Model file for the job. Use its own axes, mm. A direction names the side the tool comes from. Round coordinates to 2 decimals unless told otherwise and drop trailing zeros. Order: outer loops, then holes, each group sorted by start corner. A loop starts at its lowest first (then second) coordinate and runs counter-clockwise, first axis right, second up. Notation, with made-up numbers: (69, 15.5) - (116, 15.5) arc R38 cw to (116, 54.5) - close; hole circle Ø7 at (83, 8.25). An arc over 180 degrees is marked (long way). Answer as CSV lines item,"result". Start each with the question number.
1. Band-saw the part on D-D on z = -5.25. List the corners of the cut face in (x, y), then the cut area to 3 significant figures.
2. Band-saw the part on B-B on y = 17. List the corners of the cut face in (x, z), then the cut area to 3 significant figures.
3. Band-saw the part on C-C on y = 42. List the corners of the cut face in (x, z), then the cut area to 3 significant figures.
4. Wall check: line 1 along X through (y, z) = (2.1, 0); line 2 along Y through (x, z) = (0, 12.25); line 3 along X through (y, z) = (35, -4.5). Give the ranges that are in metal, low to high. Write a range as [from, to].
5. Pin check, flat tips, straight feed: pin 1 Ø9 at (x, y) = (25, 15) entering from +Z; pin 2 Ø1 at (x, z) = (-12.5, 9) entering from +Y; pin 3 Ø13.5 at (x, z) = (-20, 0) entering from +Y. Stop position of each tip, or through.
6. 3-axis set-ups, long thin cutter, end or side, ignore diameter. For faces 1 (the face through (-1.301, 32.143, 11.521)), 2 (the face through (-35.14, 25.35, 12.1)), 3 (the face through (-8, 3, 0)): which of +Z, -Z, +X, -X, +Y, -Y reach the whole face in a straight line?
7. Band-saw the part on A-A on z = 0. List the corners of the cut face in (x, y).
8. Pull direction Z, two halves, no side cores. Call faces 4 (the face through (0.33, 1.521, -7.493)), 5 (the face through (35.14, 25.35, -12.1)), 6 (the face through (-0.976, 27.436, 11.521)): released by +Z, released by -Z, zero draft, split by the parting line, or undercut.
```python
from build123d import *

# Parameters (mm, degrees)
SKETCH1_W                                    = 72
SKETCH1_H                                    = 26
BOSS_EXTRUDE1_DEPTH                          = 50
FILLET1_R                                    = 3
SHELL1_START                                 = -33
SHELL1_OUTLINE_W                             = 47
SHELL1_OUTLINE_H                             = 20
SHELL1_DEPTH                                 = 66
SKETCH2_R                                    = 7.5
CUT_EXTRUDE1_DEPTH                           = 61.613529843
CSK_FOR_M3_COUNTERSUNK_FLAT_HEAD_SCR_2_COUNT = 2
CSK_FOR_M3_COUNTERSUNK_FLAT_HEAD_SCR_2_PITCH = 30.663496213
CSK_FOR_M3_COUNTERSUNK_FLAT_HEAD_SCR_3_COUNT = 2
CSK_FOR_M3_COUNTERSUNK_FLAT_HEAD_SCR_3_PITCH = 30.663496213
CUT_EXTRUDE2_REACH                           = 68.873
SKETCH6_R                                    = 6
SKETCH6_R_2                                  = 7.5
SKETCH6_R_3                                  = 5


# Read off the part's stored shape, not the designer's step: Shell1
with BuildPart() as part:
    # Sketch1 → Boss-Extrude1 (new body)
    with BuildSketch(Plane(origin=(0, 0, 0), x_dir=(1, 0, 0), z_dir=(0, 1, 0))):
        Rectangle(SKETCH1_W, SKETCH1_H)
    extrude(amount=BOSS_EXTRUDE1_DEPTH)

    # Fillet1
    fillet1_edges = [part.edges().sort_by_distance(p)[0] for p in [
        (-36, 25, -13),
        (36, 25, -13),
        (36, 25, 13),
        (-36, 25, 13),
    ]]
    fillet(fillet1_edges, radius=FILLET1_R)

    # Shell1 outline → Shell1 (cut)
    with BuildSketch(Plane.YZ.offset(SHELL1_START)):
        with Locations((26.5, 0)):
            Rectangle(SHELL1_OUTLINE_W, SHELL1_OUTLINE_H)
    extrude(amount=SHELL1_DEPTH, mode=Mode.SUBTRACT)

    # Sketch2 → Cut-Extrude1 (cut, through all)
    with BuildSketch(Plane(origin=(0, 3, 0), x_dir=(1, 0, 0), z_dir=(0, 1, 0))):
        with Locations(Location((0, 0, 0), (0, 0, 270))):
            Circle(SKETCH2_R)
        with Locations(Location((-20, 0, 0), (0, 0, 270))):
            Circle(SKETCH2_R)
        with Locations(Location((20, 0, 0), (0, 0, 270))):
            Circle(SKETCH2_R)
    extrude(amount=-CUT_EXTRUDE1_DEPTH, mode=Mode.SUBTRACT)

    # Sketch4 → CSK for M3 Countersunk Flat Head Screw1 (revolve, cut)
    with BuildSketch(Plane(origin=(0, 38, -10), x_dir=(0, -1, 0), z_dir=(1, 0, 0))):
        Polygon((0, 0), (0, 3), (1.7, 3), (1.7, 1.45), (3.15, 0), align=None)
    csk_for_m3_countersunk_flat_head_screw1 = revolve(axis=Axis((0, 38, -3.65), (0, 0, -1)), mode=Mode.SUBTRACT)

    # CSK for M3 Countersunk Flat Head Scr 2: CSK for M3 Countersunk Flat Head Screw1 ×2
    with Locations(*[Vector(-0.4076508403738889, -0.9131378824375114, 0) * (i * CSK_FOR_M3_COUNTERSUNK_FLAT_HEAD_SCR_2_PITCH) for i in range(1, CSK_FOR_M3_COUNTERSUNK_FLAT_HEAD_SCR_2_COUNT)]):
        add(csk_for_m3_countersunk_flat_head_screw1, mode=Mode.SUBTRACT)

    # CSK for M3 Countersunk Flat Head Scr 3: CSK for M3 Countersunk Flat Head Screw1 ×2
    with Locations(*[Vector(0.4076508403738889, -0.9131378824375114, 0) * (i * CSK_FOR_M3_COUNTERSUNK_FLAT_HEAD_SCR_3_PITCH) for i in range(1, CSK_FOR_M3_COUNTERSUNK_FLAT_HEAD_SCR_3_COUNT)]):
        add(csk_for_m3_countersunk_flat_head_screw1, mode=Mode.SUBTRACT)

    # Sketch6 → Cut-Extrude2 (cut, up to next)
    with BuildSketch(Plane.XY.offset(13), mode=Mode.PRIVATE) as cut_extrude2_sk1:
        with Locations((0, 38)):
            Circle(SKETCH6_R)
    cut_extrude2_tool1 = extrude(cut_extrude2_sk1.sketch, amount=-CUT_EXTRUDE2_REACH, mode=Mode.PRIVATE) & part.part
    # Sketch6 → Cut-Extrude2 (cut, up to next)
    with BuildSketch(Plane.XY.offset(13), mode=Mode.PRIVATE) as cut_extrude2_sk2:
        with Locations((-12.5, 10)):
            Circle(SKETCH6_R)
    cut_extrude2_tool2 = extrude(cut_extrude2_sk2.sketch, amount=-CUT_EXTRUDE2_REACH, mode=Mode.PRIVATE) & part.part
    # Sketch6 → Cut-Extrude2 (cut, up to next)
    with BuildSketch(Plane.XY.offset(13), mode=Mode.PRIVATE) as cut_extrude2_sk3:
        with Locations((12.5, 10)):
            Circle(SKETCH6_R)
    cut_extrude2_tool3 = extrude(cut_extrude2_sk3.sketch, amount=-CUT_EXTRUDE2_REACH, mode=Mode.PRIVATE) & part.part
    # Sketch6 → Cut-Extrude2 (cut, up to next)
    with BuildSketch(Plane.XY.offset(13), mode=Mode.PRIVATE) as cut_extrude2_sk4:
        with Locations((0, 20)):
            Circle(SKETCH6_R_2)
    cut_extrude2_tool4 = extrude(cut_extrude2_sk4.sketch, amount=-CUT_EXTRUDE2_REACH, mode=Mode.PRIVATE) & part.part
    # Sketch6 → Cut-Extrude2 (cut, up to next)
    with BuildSketch(Plane.XY.offset(13), mode=Mode.PRIVATE) as cut_extrude2_sk5:
        with Locations((24, 42)):
            Circle(SKETCH6_R)
    cut_extrude2_tool5 = extrude(cut_extrude2_sk5.sketch, amount=-CUT_EXTRUDE2_REACH, mode=Mode.PRIVATE) & part.part
    # Sketch6 → Cut-Extrude2 (cut, up to next)
    with BuildSketch(Plane.XY.offset(13), mode=Mode.PRIVATE) as cut_extrude2_sk6:
        with Locations((16, 28)):
            Circle(SKETCH6_R_2)
    cut_extrude2_tool6 = extrude(cut_extrude2_sk6.sketch, amount=-CUT_EXTRUDE2_REACH, mode=Mode.PRIVATE) & part.part
    # Sketch6 → Cut-Extrude2 (cut, up to next)
    with BuildSketch(Plane.XY.offset(13), mode=Mode.PRIVATE) as cut_extrude2_sk7:
        with Locations((-16, 28)):
            Circle(SKETCH6_R_2)
    cut_extrude2_tool7 = extrude(cut_extrude2_sk7.sketch, amount=-CUT_EXTRUDE2_REACH, mode=Mode.PRIVATE) & part.part
    # Sketch6 → Cut-Extrude2 (cut, up to next)
    with BuildSketch(Plane.XY.offset(13), mode=Mode.PRIVATE) as cut_extrude2_sk8:
        with Locations((-24, 42)):
            Circle(SKETCH6_R)
    cut_extrude2_tool8 = extrude(cut_extrude2_sk8.sketch, amount=-CUT_EXTRUDE2_REACH, mode=Mode.PRIVATE) & part.part
    # Sketch6 → Cut-Extrude2 (cut, up to next)
    with BuildSketch(Plane.XY.offset(13), mode=Mode.PRIVATE) as cut_extrude2_sk9:
        with Locations((25, 15)):
            Circle(SKETCH6_R_3)
    cut_extrude2_tool9 = extrude(cut_extrude2_sk9.sketch, amount=-CUT_EXTRUDE2_REACH, mode=Mode.PRIVATE) & part.part
    # Sketch6 → Cut-Extrude2 (cut, up to next)
    with BuildSketch(Plane.XY.offset(13), mode=Mode.PRIVATE) as cut_extrude2_sk10:
        with Locations((-25, 15)):
            Circle(SKETCH6_R_3)
    cut_extrude2_tool10 = extrude(cut_extrude2_sk10.sketch, amount=-CUT_EXTRUDE2_REACH, mode=Mode.PRIVATE) & part.part
    add(cut_extrude2_tool1.solids().sort_by_distance((0, 38, 13))[0], mode=Mode.SUBTRACT)
    add(cut_extrude2_tool2.solids().sort_by_distance((-12.5, 10, 13))[0], mode=Mode.SUBTRACT)
    add(cut_extrude2_tool3.solids().sort_by_distance((12.5, 10, 13))[0], mode=Mode.SUBTRACT)
    add(cut_extrude2_tool4.solids().sort_by_distance((0, 20, 13))[0], mode=Mode.SUBTRACT)
    add(cut_extrude2_tool5.solids().sort_by_distance((24, 42, 13))[0], mode=Mode.SUBTRACT)
    add(cut_extrude2_tool6.solids().sort_by_distance((16, 28, 13))[0], mode=Mode.SUBTRACT)
    add(cut_extrude2_tool7.solids().sort_by_distance((-16, 28, 13))[0], mode=Mode.SUBTRACT)
    add(cut_extrude2_tool8.solids().sort_by_distance((-24, 42, 13))[0], mode=Mode.SUBTRACT)
    add(cut_extrude2_tool9.solids().sort_by_distance((25, 15, 13))[0], mode=Mode.SUBTRACT)
    add(cut_extrude2_tool10.solids().sort_by_distance((-25, 15, 13))[0], mode=Mode.SUBTRACT)


solid = part.part
```
Reply:
1,outline,"(-36, 0) - (-25.36, 0) - (-25.36, 3) - (-33, 3) - (-33, 50) - (-36, 50) - close; (-14.64, 0) - (-5.36, 0) - (-5.36, 3) - (-14.64, 3) - close; (5.36, 0) - (14.64, 0) - (14.64, 3) - (5.36, 3) - close; (25.36, 0) - (36, 0) - (36, 50) - (33, 50) - (33, 3) - (25.36, 3) - close"
1,area,"402 mm2"
2,outline,"(-36, -10) arc R3 ccw to (-33, -13) - (33, -13) arc R3 ccw to (36, -10) - (36, 10) arc R3 ccw to (33, 13) - (29.58, 13) - (29.58, 10) - (33, 10) - (33, -10) - (-33, -10) - (-33, 10) - (-29.58, 10) - (-29.58, 13) - (-33, 13) arc R3 ccw to (-36, 10) - close; (-20.42, 10) - (-6.87, 10) - (-6.87, 13) - (-20.42, 13) - close; (6.87, 10) - (20.42, 10) - (20.42, 13) - (6.87, 13) - close"
2,area,"448 mm2"
3,outline,"(-36, -10) arc R3 ccw to (-33, -13) - (33, -13) arc R3 ccw to (36, -10) - (36, 10) arc R3 ccw to (33, 13) - (30, 13) - (30, 10) - (33, 10) - (33, -10) - (-33, -10) - (-33, 10) - (-30, 10) - (-30, 13) - (-33, 13) arc R3 ccw to (-36, 10) - close; (-18, 10) - (-4.47, 10) - (-4.47, 13) - (-18, 13) - close; (4.47, 10) - (18, 10) - (18, 13) - (4.47, 13) - close"
3,area,"445 mm2"
4,line 1,"x = [-36, -27.5], [-12.5, -7.5], [7.5, 12.5], [27.5, 36]"
4,line 2,"y = [0, 12.5], [27.5, 32], [44, 50]"
4,line 3,"x = [-36, -33], [33, 36]"
5,pin 1,"stops at z = -10"
5,pin 2,"stops at y = 3"
5,pin 3,"passes through"
6,face 1,"+Z"
6,face 2,"+Z, -X, +Y, -Y"
6,face 3,"+Y"
7,outline,"(-36, 0) - (-27.5, 0) - (-27.5, 3) - (-33, 3) - (-33, 50) - (-36, 50) - close; (-12.5, 0) - (-7.5, 0) - (-7.5, 3) - (-12.5, 3) - close; (7.5, 0) - (12.5, 0) - (12.5, 3) - (7.5, 3) - close; (27.5, 0) - (36, 0) - (36, 50) - (33, 50) - (33, 3) - (27.5, 3) - close"
8,face 4,"undercut"
8,face 5,"released by -Z"
8,face 6,"zero draft"
